Work out the finished part from the listing and answer in its coordinate system (mm). Give positions to 0.01 mm unless a question says otherwise; leave off trailing zeros. Write each loop counter-clockwise with the first axis right and the second up, starting at its lowest first coordinate (ties: lowest second). Pieces come first, ordered by that corner, then holes. Notation, with made-up numbers: (59, -4.75) - (102, -4.75) arc R24 cw to (102, 28.25) - close; hole circle Ø3 at (59, 28). An arc over 180 degrees is marked (long way). Write item = value, one per line.
Autodesk Inventor part; units mm, degrees
ref_plane "YZ Plane" through (0, 0, 0) normal (1, 0, 0) x (0, 1, 0)
ref_plane "XZ Plane" through (0, 0, 0) normal (0, 1, 0) x (-1, 0, 0)
ref_plane "XY Plane" through (0, 0, 0) normal (0, 0, 1) x (1, 0, 0)
sketch "Boceto1" plane through (0, 0, 0) normal (1, 0, 0) x (0, 1, 0)
  line L0 (7.6041, 11.4062) -> (-8.6387, 11.4062)
  line L1 (-8.6387, 11.4062) -> (-8.6387, -13.3718)
  line L2 (-8.6387, -13.3718) -> (7.6041, -13.3718)
  line L3 (7.6041, -13.3718) -> (7.6041, 11.4062)
  point P0 (0, 0)
extrude "Extrusión1" add sketch "Boceto1" along normal blind 10
sketch "Boceto2" plane through (10, 0, 0) normal (1, 0, 0) x (0, 0, -1)
  line L0 (13.3718, -8.6387) -> (13.3718, 7.6041)
  line L1 (-11.4062, -8.6387) -> (13.3718, -8.6387)
  point P0 (0, 0)
  point P1 (0.575, 6.3613)
  point P2 (13.3718, -0.5173)
  dimension "d9" = 12.7969
  dimension "d10" = 15
hole "Agujero1" at (10, 6.3613, -0.575) direction (-1, 0, 0) diameter 4.134 end through all
equation "\"Radio_pliegue\" = Grosor"
equation "\"Anchura_desahogo_plegado\" = Grosor"
equation "\"Profundidad_desahogo_plegado\" = 0.5 * Grosor"
equation "\"Tamaño_destalonado\" = 4 * Grosor"
equation "\"Remanente_mínimo\" = 2 * Grosor"
equation "\"Radiodetransición\" = Radio_pliegue"
equation "\"Tamaño_de_radio_de_Jacobi\" = Radio_pliegue"
equation "\"TamañoSeparación\" = Grosor"
properties part number "Proyecto 1"
1. For a pull along Y with two mould halves and no side action, classify faces 1 (the flat face through (5, -8.639, -1)), 2 (the flat face through (10, -1, -1)), 3 (the flat face through (5, 7.604, -8)), 4 (the cylindrical face through (4.93, 4.295, -0.639)) as pulls with the +Y half, pulls with the -Y half, needs draft (parallel to the pull), parting line crosses it, or undercut.
Solution:
face_1 = pulls with the -Y half
face_2 = needs draft
face_3 = pulls with the +Y half
face_4 = undercut
2. Straight lines are drawn through the part: line 1 (Z direction, x = 6, y = 5.5); line 2 (Z direction, x = 9.25, y = 4.5); line 3 (Y direction, x = 6.5, z = -1.75). For each, find the intervals that lie inside material, in ascending order.
Solution:
line_1 = -13.37 to -2.45, 1.3 to 11.41
line_2 = -13.37 to -1.47, 0.32 to 11.41
line_3 = -8.64 to 4.66
3. Find section B-B, the plane x = 3.75. Give the vertices of the cut face in (y, z) (3 decimals), then the cut area to 3 significant figures.
Solution:
outline = (-8.639, -13.372) - (7.604, -13.372) - (7.604, -2.227) arc R2.067 cw (long way) to (7.604, 1.077) - (7.604, 11.406) - (-8.639, 11.406) - close
area = 391 mm^2
4. Find section A-A, the plane y = 6. Give the vertices of the cut face in (x, z).
Solution:
outline = (0, -13.37) - (10, -13.37) - (10, -2.61) - (0, -2.61) - close; (0, 1.46) - (10, 1.46) - (10, 11.41) - (0, 11.41) - close
